Source: CAD feature listing. Evaluate the final solid. Frame: model axes, mm. A direction names the side the tool comes from. Coordinates: 2 decimals unless noted, no trailing zeros. Order: outer loops, then holes, each group sorted by start corner. A loop starts at its lowest first (then second) coordinate and runs counter-clockwise, first axis right, second up.
Item 1: Contact query for flat-ended pins moving along their axis: P1, Ø8, axis at x = 41, y = 0, coming from the +Z side; P2, Ø12, axis at x = 39, y = -8.5, coming from the +Z side. Output: stop coordinate, or through.
Item 2: Section B-B on x = 19. Return the cut outline in (y, z).
Item 3: Section D-D on z = 20.5. Return the cut outline in (x, y), then the cut area to 3 significant figures.
Item 4: Ray query, line 1 (X direction, y = 1.5, z = 35); line 2 (X direction, y = 5, z = 60.5); line 3 (Y direction, x = 55, z = 46). Return the intervals inside material, ascending.
Item 5: Mould query, pull axis X, two halves, no side actions, for faces 4 (the flat face through (63.5, 0, 31)), 5 (the flat face through (-3, -13.97, 28)), 6 (the flat face through (-25.4, 0, 34)), 7 (the flat face through (-1, -19.05, 31)). Classes: released by +X, released by -X, zero draft, split by the parting line, or undercut.
Item 6: Section A-A on z = 55.5. Return the cut outline in (x, y).
Item 7: Section C-C on y = 5. Return the cut outline in (x, z).
Item 8: Reachability of faces 1 (the flat face through (30.48, 0, 34)), 2 (the flat face through (-63.5, 0, 31)), 3 (the flat face through (1.8, 14.2, 50.8)) from +Z, -Z, +X, -X, +Y, -Y: full face, straight path, thin tool, end or side. Return the list, or none.
from build123d import *

# Parameters (mm, degrees)
F0_W      = 38.1
F0_H      = 38.1
F1_DEPTH  = 63.5
F2_T      = -5.08
F0_W_2    = 50.8
F3_DEPTH  = 50.8
F0_W_3    = 33.02
F4_DEPTH  = 63.5
F5_T      = -5.08
F0_W_4    = 5.08
F7_DEPTH  = 63.5
F8_DEPTH  = 63.5
F9_T      = -5.08
F10_DEPTH = 50.8


# Not quite as in the source:
# - a shell that OpenCascade refuses in one call is made with other operations: the cavity is built on its own and cut out


with BuildPart() as f1:
    # F0 (on Top) → F1 (new body)
    with BuildSketch(Plane.XY):
        with Locations((-44.45, 0)):
            Rectangle(F0_W, F0_H)
    extrude(amount=F1_DEPTH)

    # F2
    f2_openings = [f1.faces().sort_by_distance(p)[0] for p in [
        (-44.45, 0, 63.5),
    ]]
    offset(amount=F2_T, openings=f2_openings)

    # F0 (on Top) → F3 (join)
    with BuildSketch(Plane.XY):
        Rectangle(F0_W_2, F0_H)
    extrude(amount=F3_DEPTH)

    # F5: a shell. OpenCascade refuses it in one call, so the cavity is built on its own and cut out:
    # the body offset inwards by the wall thickness, plus a prism from it out through each open face.
    f5_core = offset(f1.part, amount=F5_T, kind=Kind.INTERSECTION, mode=Mode.PRIVATE)
    f5_exits = [f5_core.faces().sort_by_distance(p)[0] for p in [
        (-2.54, 0, 45.72),
    ]]
    add(f5_core, mode=Mode.SUBTRACT)
    extrude(f5_exits, amount=-F5_T, mode=Mode.SUBTRACT)

    # F0 (on Top) → F7 (join)
    with BuildSketch(Plane.XY):
        with Locations((27.94, 0)):
            Rectangle(F0_W_4, F0_H)
    extrude(amount=F7_DEPTH)

    # F0 (on Top) → F8 (join)
    with BuildSketch(Plane.XY):
        with Locations((46.99, 0)):
            Rectangle(F0_W_3, F0_H)
    extrude(amount=F8_DEPTH)

    # F9: a shell. OpenCascade refuses it in one call, so the cavity is built on its own and cut out:
    # the body offset inwards by the wall thickness, plus a prism from it out through each open face.
    f9_core = offset(f1.part, amount=F9_T, kind=Kind.INTERSECTION, mode=Mode.PRIVATE)
    f9_exits = [f9_core.faces().sort_by_distance(p)[0] for p in [
        (44.45, 0, 58.42),
    ]]
    add(f9_core, mode=Mode.SUBTRACT)
    extrude(f9_exits, amount=-F9_T, mode=Mode.SUBTRACT)

    # F0 (on Top) → F10 (join)
    with BuildSketch(Plane.XY):
        with Locations((27.94, 0)):
            Rectangle(F0_W_4, F0_H)
    extrude(amount=F10_DEPTH)


with BuildPart() as f4:
    # F0 (on Top) → F4 (new body)
    with BuildSketch(Plane.XY):
        with Locations((46.99, 0)):
            Rectangle(F0_W_3, F0_H)
    extrude(amount=F4_DEPTH)


solid = f1.part
Answer list:
1. P1: stops at z = 5.08
1. P2: stops at z = 63.5
2. outline: (-19.05, 0) - (19.05, 0) - (19.05, 50.8) - (13.97, 50.8) - (13.97, 5.08) - (-13.97, 5.08) - (-13.97, 50.8) - (-19.05, 50.8) - close
3. outline: (-63.5, -19.05) - (63.5, -19.05) - (63.5, 19.05) - (-63.5, 19.05) - close; hole (-58.42, -13.97) - (-30.48, -13.97) - (-30.48, 13.97) - (-58.42, 13.97) - close; hole (-25.4, -13.97) - (20.32, -13.97) - (20.32, 13.97) - (-25.4, 13.97) - close; hole (30.48, -13.97) - (58.42, -13.97) - (58.42, 13.97) - (30.48, 13.97) - close
3. area: 2,000 mm2
4. line 1: x = -63.5 to -58.42, -30.48 to -25.4, 20.32 to 30.48, 58.42 to 63.5
4. line 2: x = -63.5 to -58.42, -30.48 to -25.4, 25.4 to 30.48, 58.42 to 63.5
4. line 3: y = -19.05 to -13.97, 13.97 to 19.05
5. face 4: released by +X
5. face 5: undercut
5. face 6: undercut
5. face 7: zero draft
6. outline: (-63.5, -19.05) - (-25.4, -19.05) - (-25.4, 19.05) - (-63.5, 19.05) - close; (25.4, -19.05) - (63.5, -19.05) - (63.5, 19.05) - (25.4, 19.05) - close; hole (-58.42, -13.97) - (-30.48, -13.97) - (-30.48, 13.97) - (-58.42, 13.97) - close; hole (30.48, -13.97) - (58.42, -13.97) - (58.42, 13.97) - (30.48, 13.97) - close
7. outline: (-63.5, 0) - (63.5, 0) - (63.5, 63.5) - (58.42, 63.5) - (58.42, 5.08) - (30.48, 5.08) - (30.48, 63.5) - (25.4, 63.5) - (25.4, 50.8) - (20.32, 50.8) - (20.32, 5.08) - (-25.4, 5.08) - (-25.4, 63.5) - (-30.48, 63.5) - (-30.48, 5.08) - (-58.42, 5.08) - (-58.42, 63.5) - (-63.5, 63.5) - close
8. face 1: +Z
8. face 2: +Z, -Z, -X, +Y, -Y
8. face 3: +Z, +Y, -Y
